The model under review builds one solid part; all positions refer to its coordinate system, in mm. Face numbers are marked on the shaded views. A direction names the side the tool comes from. Give positions to 0.01 mm unless a question says otherwise; leave off trailing zeros. Loops run counter-clockwise (first coordinate to the right, second up) from the corner with the lowest first, then second, coordinate; pieces in that order, holes last. Notation, with made-up numbers: M -16,-34 L -1,-34 A17 cw -1,-18 Z; hole C 46,74 d4. An arc over 180 degrees is marked long. Write item = value, one per line. Start each with the question number.
1. For the marked faces 1, 2 and 3, list the 3-axis set-ups (+Z, -Z, +X, -X, +Y, -Y) from which the entire face can be reached by the end or side of a thin tool; tool diameter is ignored.
2. We need section A-A on x = 12.7. Give the boundary of the cut face in (y, z), then the cut area to 3 significant figures.
3. We need section B-B on y = -2. Give the boundary of the cut face in (x, z), then the cut area to 3 significant figures.
4. We need section C-C on z = 22. Give the boundary of the cut face in (x, y), then the cut area to 3 significant figures.
5. For pin 1 (12 mm diameter, centred on x = 57.5, z = 5.5, fed in from +Y); pin 2 (2 mm diameter, centred on x = 80, y = 4, fed in from -Z); pin 3 (2 mm diameter, centred on x = 38.5, z = 7, fed in from -Y); pin 4 (3 mm diameter, centred on x = 30.5, y = -1, fed in from +Z), all flat-tipped, find the tip position at first contact; note any pin that passes through.
6. We need section D-D on z = 12. Give the boundary of the cut face in (x, y), then the cut area to 3 significant figures.
7. Wall thickness on line 1 along Z through (x, y) = (88, -1); line 2 along Z through (x, y) = (86.5, 1.5); line 3 along Y through (x, z) = (52.5, 17): over which ranges is each line inside the solid? List them lowest first. Write a range as from..to.
from build123d import *

# Parameters (mm, degrees)
F0_W         = 12.7
F0_H         = 12.7
F1_DEPTH     = 101.6
F2_R         = 2.54
F3_DEPTH     = 25.4
F4_DEPTH     = 12.7
F5_T4_DEPTH  = 133.35
F5_S5_R      = 2.54
F5_T6_DEPTH  = 68
F5_T10_DEPTH = 133.35
F5_S11_R     = 2.54
F5_T12_DEPTH = 68
F5_T16_DEPTH = 133.35
F5_S17_R     = 2.54
F5_T18_DEPTH = 68
F5_T22_DEPTH = 133.35
F5_S23_R     = 2.54
F5_T24_DEPTH = 68


# Not quite as in the source:
# - a fillet or chamfer that OpenCascade refuses, or shapes differently, is made with other operations: its cross-section is extruded or revolved along the edge and cut away or added


with BuildPart() as f1:
    # F0 (on Right) → F1 (new body)
    with BuildSketch(Plane.YZ):
        with Locations((-1.0797850298, 14.7537575103)):
            Rectangle(F0_W, F0_H)
    extrude(amount=F1_DEPTH)

    # F2 (on face) → F3 (join)
    with BuildSketch(Plane.XY.offset(21.1037575103)):
        with Locations((12.7, -1.0797850298)):
            Circle(F2_R)
    extrude(amount=-F3_DEPTH)

    # F2 (on face) → F4 (join)
    with BuildSketch(Plane.XY.offset(21.1037575103)):
        with Locations((12.7, -1.0797850298)):
            Circle(F2_R)
    extrude(amount=F4_DEPTH)

    # F5: fillet of radius 6.35 on 4 edges, made by hand


with BuildPart() as f5_tool2:
    # F5_s3 → F5_t4 (new body)
    with BuildSketch(Plane.YZ.offset(-15.875)):
        with BuildLine():
            ThreePointArc((-7.4297850298, 14.7537575103), (-5.5699130903, 19.2438855709), (-1.0797850298, 21.1037575103))
            Line((-1.0797850298, 21.1037575103), (-7.4297850298, 21.1037575103))
            Line((-7.4297850298, 21.1037575103), (-7.4297850298, 14.7537575103))
        make_face()
    extrude(amount=F5_T4_DEPTH)

    # F5_s5 → F5_t6 (cut, symmetric)
    with BuildSketch(Plane.XY.offset(17.9)):
        with Locations((12.7, -1.0797850298)):
            Circle(F5_S5_R)
    extrude(amount=F5_T6_DEPTH, both=True, mode=Mode.SUBTRACT)


with BuildPart() as f1_1:
    add(f1.part)

    # F5_t1: cut F5_tool2
    add(f5_tool2.part, mode=Mode.SUBTRACT)


with BuildPart() as f5_tool8:
    # F5_s9 → F5_t10 (new body)
    with BuildSketch(Plane.YZ.offset(-15.875)):
        with BuildLine():
            ThreePointArc((-1.0797850298, 21.1037575103), (3.4103430308, 19.2438855709), (5.2702149702, 14.7537575103))
            Line((5.2702149702, 14.7537575103), (5.2702149702, 21.1037575103))
            Line((5.2702149702, 21.1037575103), (-1.0797850298, 21.1037575103))
        make_face()
    extrude(amount=F5_T10_DEPTH)

    # F5_s11 → F5_t12 (cut, symmetric)
    with BuildSketch(Plane.XY.offset(17.9)):
        with Locations((12.7, -1.0797850298)):
            Circle(F5_S11_R)
    extrude(amount=F5_T12_DEPTH, both=True, mode=Mode.SUBTRACT)


with BuildPart() as f1_2:
    add(f1_1.part)

    # F5_t7: cut F5_tool8
    add(f5_tool8.part, mode=Mode.SUBTRACT)


with BuildPart() as f5_tool14:
    # F5_s15 → F5_t16 (new body)
    with BuildSketch(Plane.YZ.offset(-15.875)):
        with BuildLine():
            ThreePointArc((-7.4297850298, 14.7537575103), (-5.5699130903, 10.2636294498), (-1.0797850298, 8.4037575103))
            Line((-1.0797850298, 8.4037575103), (-7.4297850298, 8.4037575103))
            Line((-7.4297850298, 8.4037575103), (-7.4297850298, 14.7537575103))
        make_face()
    extrude(amount=F5_T16_DEPTH)

    # F5_s17 → F5_t18 (cut, symmetric)
    with BuildSketch(Plane.XY.offset(11.6)):
        with Locations((12.7, -1.0797850298)):
            Circle(F5_S17_R)
    extrude(amount=F5_T18_DEPTH, both=True, mode=Mode.SUBTRACT)


with BuildPart() as f1_3:
    add(f1_2.part)

    # F5_t13: cut F5_tool14
    add(f5_tool14.part, mode=Mode.SUBTRACT)


with BuildPart() as f5_tool20:
    # F5_s21 → F5_t22 (new body)
    with BuildSketch(Plane.YZ.offset(-15.875)):
        with BuildLine():
            ThreePointArc((-1.0797850298, 8.4037575103), (3.4103430308, 10.2636294498), (5.2702149702, 14.7537575103))
            Line((5.2702149702, 14.7537575103), (5.2702149702, 8.4037575103))
            Line((5.2702149702, 8.4037575103), (-1.0797850298, 8.4037575103))
        make_face()
    extrude(amount=F5_T22_DEPTH)

    # F5_s23 → F5_t24 (cut, symmetric)
    with BuildSketch(Plane.XY.offset(11.6)):
        with Locations((12.7, -1.0797850298)):
            Circle(F5_S23_R)
    extrude(amount=F5_T24_DEPTH, both=True, mode=Mode.SUBTRACT)


with BuildPart() as f1_4:
    add(f1_3.part)

    # F5_t19: cut F5_tool20
    add(f5_tool20.part, mode=Mode.SUBTRACT)


solid = f1_4.part
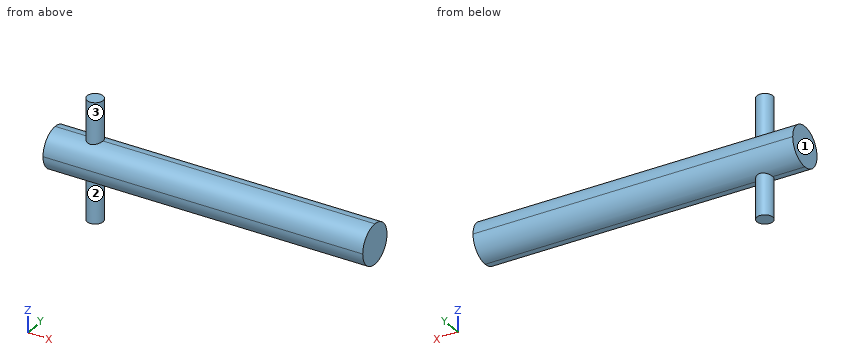
Final values:
q1.face_1 = +Z, -Z, -X, +Y, -Y
q1.face_2 = -Z
q1.face_3 = +Z
q2.outline = M -3.62,-4.3 L 1.46,-4.3 L 1.46,8.93 A6.35 ccw 1.46,20.57 L 1.46,33.8 L -3.62,33.8 L -3.62,20.57 A6.35 ccw -3.62,8.93 Z
q2.area = 257 mm²
q3.outline = M 0,8.47 L 10.33,8.47 L 10.33,-4.3 L 15.07,-4.3 L 15.07,8.47 L 101.6,8.47 L 101.6,21.04 L 15.07,21.04 L 15.07,33.8 L 10.33,33.8 L 10.33,21.04 L 0,21.04 Z
q3.area = 1,400 mm²
q4.outline = C 12.7,-1.08 d5.08
q4.area = 20.3 mm²
q5.pin_1 = 4.37
q5.pin_2 = 9.89
q5.pin_3 = through
q5.pin_4 = 21.1
q6.outline = M 0,-6.8 L 101.6,-6.8 L 101.6,4.64 L 0,4.64 Z
q6.area = 1,160 mm²
q7.line_1 = 8.4..21.1
q7.line_2 = 8.95..20.56
q7.line_3 = -7.02..4.86
